from build123d import *

# Parameters (mm, degrees)
EXTRUSION2_DEPTH = 12.7


with BuildPart() as part:
    # Sketch1 → Extrusion2 (new body)
    with BuildSketch(Plane.XY):
        with BuildLine():
            Line((15.584253212, 20.907446686), (10.543218779, 15.866412253))
            ThreePointArc((10.543218779, 15.866412253), (7.93326935, 17.319518972), (5.128249951, 18.346758636))
            Line((5.128249951, 18.346758636), (5.128249951, 25.803528454))
            Line((5.128249951, 25.803528454), (-3.764066203, 25.803528454))
            Line((-3.764066203, 25.803528454), (-3.764066203, 18.674429191))
            ThreePointArc((-3.764066203, 18.674429191), (-6.637080757, 17.856417866), (-9.346897128, 16.59933776))
            Line((-9.346897128, 16.59933776), (-14.619629632, 21.872070265))
            Line((-14.619629632, 21.872070265), (-20.907446686, 15.584253212))
            Line((-20.907446686, 15.584253212), (-15.866412253, 10.543218779))
            ThreePointArc((-15.866412253, 10.543218779), (-17.319518972, 7.93326935), (-18.346758636, 5.128249951))
            Line((-18.346758636, 5.128249951), (-25.803528454, 5.128249951))
            Line((-25.803528454, 5.128249951), (-25.803528454, -3.764066203))
            Line((-25.803528454, -3.764066203), (-18.674429191, -3.764066203))
            ThreePointArc((-18.674429191, -3.764066203), (-17.856417866, -6.637080757), (-16.59933776, -9.346897128))
            Line((-16.59933776, -9.346897128), (-21.872070265, -14.619629632))
            Line((-21.872070265, -14.619629632), (-15.584253212, -20.907446686))
            Line((-15.584253212, -20.907446686), (-10.543218779, -15.866412253))
            ThreePointArc((-10.543218779, -15.866412253), (-7.93326935, -17.319518972), (-5.128249951, -18.346758636))
            Line((-5.128249951, -18.346758636), (-5.128249951, -25.803528454))
            Line((-5.128249951, -25.803528454), (3.764066203, -25.803528454))
            Line((3.764066203, -25.803528454), (3.764066203, -18.674429191))
            ThreePointArc((3.764066203, -18.674429191), (6.637080757, -17.856417866), (9.346897128, -16.59933776))
            Line((9.346897128, -16.59933776), (14.619629632, -21.872070265))
            Line((14.619629632, -21.872070265), (20.907446686, -15.584253212))
            Line((20.907446686, -15.584253212), (15.866412253, -10.543218779))
            ThreePointArc((15.866412253, -10.543218779), (17.319518972, -7.93326935), (18.346758636, -5.128249951))
            Line((18.346758636, -5.128249951), (25.803528454, -5.128249951))
            Line((25.803528454, -5.128249951), (25.803528454, 3.764066203))
            Line((25.803528454, 3.764066203), (18.674429191, 3.764066203))
            ThreePointArc((18.674429191, 3.764066203), (17.856417866, 6.637080757), (16.59933776, 9.346897128))
            Line((16.59933776, 9.346897128), (21.872070265, 14.619629632))
            Line((21.872070265, 14.619629632), (15.584253212, 20.907446686))
        make_face()
        with BuildLine():
            ThreePointArc((-3.116590945, 0.606206137), (-2.754939335, -1.578269388), (-1.053419361, -2.995151524))
            Line((-1.053419361, -2.995151524), (-1.053419361, -4.468974981))
            Line((-1.053419361, -4.468974981), (1.033305558, -4.468974981))
            Line((1.033305558, -4.468974981), (1.033305558, -3.00215))
            ThreePointArc((1.033305558, -3.00215), (2.744291052, -1.596712756), (3.120586988, 0.585287835))
            Line((3.120586988, 0.585287835), (4.396955543, 1.322199563))
            Line((4.396955543, 1.322199563), (3.353593084, 3.129356353))
            Line((3.353593084, 3.129356353), (2.083285387, 2.395943863))
            ThreePointArc((2.083285387, 2.395943863), (0.010648283, 3.174982144), (-2.067167627, 2.409863689))
            Line((-2.067167627, 2.409863689), (-3.343536182, 3.146775418))
            Line((-3.343536182, 3.146775418), (-4.386898641, 1.339618628))
            Line((-4.386898641, 1.339618628), (-3.116590945, 0.606206137))
        make_face(mode=Mode.SUBTRACT)
    extrude(amount=EXTRUSION2_DEPTH)


solid = part.part
Input: part model. Units: mm. Frame: model coordinates. A direction names the side the tool comes from. Give positions to 0.01 mm unless a question says otherwise; leave off trailing zeros. Order: outer loops, then holes, each group sorted by start corner. A loop starts at its lowest first (then second) coordinate and runs counter-clockwise, first axis right, second up. Notation, with made-up numbers: (-33.5, 47.5) -> (-19.5, 47.5) arc R21 ccw to (-19.5, 74.5) -> close; hole circle Ø1 at (-35, -22.75). An arc over 180 degrees is marked (long way). Use one line per item in the form item = value.
1) Line query: probe 1 along Y at (x, z) = (19, 1.5); probe 2 along Y at (x, z) = (19.5, 12); probe 3 along X at (y, z) = (2.5, 10.25). Output: solid intervals per line, ascending.
Response values:
probe_1 = -17.49 to -13.68, -5.13 to 3.76, 11.75 to 17.49
probe_2 = -16.99 to -14.18, -5.13 to 3.76, 12.25 to 16.99
probe_3 = -25.8 to -3.72, -2.22 to -1.96, 1.96 to 2.26, 3.72 to 25.8
2) Section A-A, the plane x = 0. Return loops of the section in (y, z) (3 decimals).
Response values:
outline = (-25.804, 0) -> (-4.469, 0) -> (-4.469, 12.7) -> (-25.804, 12.7) -> close; (3.175, 0) -> (25.804, 0) -> (25.804, 12.7) -> (3.175, 12.7) -> close
3) Section B-B, the plane x = 19.5. Return loops of the section in (y, z).
Response values:
outline = (-16.99, 0) -> (-14.18, 0) -> (-14.18, 12.7) -> (-16.99, 12.7) -> close; (-5.13, 0) -> (3.76, 0) -> (3.76, 12.7) -> (-5.13, 12.7) -> close; (12.25, 0) -> (16.99, 0) -> (16.99, 12.7) -> (12.25, 12.7) -> close
4) Section D-D, the plane x = 8.5. Return loops of the section in (y, z), and give its area (3 significant figures).
Response values:
outline = (-17.05, 0) -> (17.05, 0) -> (17.05, 12.7) -> (-17.05, 12.7) -> close
area = 433 mm^2
5) First-contact query: pin 1 Ø5 at (y, z) = (17, 4.5) entering from -X; pin 2 Ø3.5 at (x, z) = (21, 6) entering from -Y; pin 3 Ø2 at (y, z) = (22.5, 8.5) entering from +X. Flat tips, straight axial feed; report the tip coordinate or a pass-through.
Response values:
pin_1 = -20.91
pin_2 = -17.24
pin_3 = 5.13
6) Mould query, pull axis Y, two halves, no side actions, for faces 1 (the flat face through (18.422, -13.099, 6.261)), 2 (the cylindrical face through (-17.87, -6.6, 6.26)), 3 (the cylindrical face through (-7.971, -17.302, 6.261)), 4 (the flat face through (-5.128, -22, 6)). Classes: pulls with the +Y half, pulls with the -Y half, needs draft (parallel to the pull), parting line crosses it, or undercut.
Response values:
face_1 = undercut
face_2 = undercut
face_3 = pulls with the -Y half
face_4 = needs draft
7) Reachability of faces 5 (the cylindrical face through (7.971, 17.302, 6.261)), 6 (the flat face through (-18.422, 13.099, 6.261)), 7 (the flat face through (0, -4.469, 6)), 8 (the flat face through (19.2, 11.95, 6.26)) from +Z, -Z, +X, -X, +Y, -Y: full face, straight path, thin tool, end or side. Return the list, or none.
Response values:
face_5 = +Z, -Z, +Y
face_6 = +Z, -Z, -X
face_7 = +Z, -Z
face_8 = +Z, -Z, +X
8) Section C-C, the plane y = 23. Return loops of the section in (x, z).
Response values:
outline = (-3.76, 0) -> (5.13, 0) -> (5.13, 12.7) -> (-3.76, 12.7) -> close
